Read the model definition and answer for the solid it produces. Units are mm, in the model's axes. A direction names the side the tool comes from. Coordinates: 2 decimals unless noted, no trailing zeros. Order: outer loops, then holes, each group sorted by start corner. A loop starts at its lowest first (then second) coordinate and runs counter-clockwise, first axis right, second up. Notation, with made-up numbers: M 59.25,11 L 91.25,11 A24 ccw 91.25,41 Z; hole C -4,43 d6. An arc over 180 degrees is marked long. One line per question, with ' | ' between items. Start each with the question number.
1) Find section C-C, the plane y = -2. Write down the section's boundary in (x, z).
2) Consider probe 1 along X at (y, z) = (2.5, 0); probe 2 along Y at (x, z) = (0, 0.25); probe 3 along Y at (x, z) = (2.5, 2.25). Determine where each line is inside the solid, lowest interval first.
3) The mould has two halves that part along X. Classify faces 1 (the face through (1, 11.79, -1)), 2 (the face through (0, 11, -2.5)), 3 (the face through (1.151, 9.459, -1.502)): +X half, -X half, draft (parallel to the pull), parting line (faces both ways), or undercut.
4) Given P1, Ø1.6, axis at y = 10.5, z = 1, coming from the -X side; P2, Ø2, axis at x = 0.5, y = 4.5, coming from the -Z side; P3, Ø3, axis at x = 0.5, z = 2, coming from the +Y side; P4, Ø1.3, axis at x = 0, y = 11, coming from the -Z side, each flat-ended and moving along its own axis, determine where each tip first touches the part or whether it passes through.
5) Find section A-A, the plane x = 0. Write down the section's boundary in (y, z), plus the area to 3 significant figures.
6) A tool of negligible diameter and unlimited length cuts with its end or side. For faces 4 (the face through (-0.6, 11, -2)), 5 (the face through (0, -18.01, 0)), 6 (the face through (-0.541, -4.349, 1.717)), from which of +Z, -Z, +X, -X, +Y, -Y can it reach the whole face along a straight path? Write none if from no direction.
7) Find section B-B, the plane z = 0. Write down the section's boundary in (x, y), plus the area to 3 significant figures.
from build123d import *

# Parameters (mm, degrees)
CUT_EXTRUDE1_DEPTH = 1.43


with BuildPart() as part:
    # Sketch1 → Revolve1 (revolve)
    with BuildSketch(Plane(origin=(0, 0, 0), x_dir=(0, 0, -1), z_dir=(1, 0, 0))):
        Polygon((0, 11.789679649), (-3.7, 11.789679649), (-1.8, 9.339679649), (-1.8, -17.660320351), (-1.528571429, -18.010320351), (0, -18.010320351), align=None)
    revolve(axis=Axis((0, 14.440515102, 0), (0, -1, 0)))

    # Sketch2 → Cut-Extrude1 (cut)
    with BuildSketch(Plane(origin=(0, 11.789679649, 0), x_dir=(1, 0, 0), z_dir=(0, 1, 0))):
        Polygon((2.5, -0.6), (0.6, -0.6), (0.6, -2.5), (-0.6, -2.5), (-0.6, -0.6), (-2.5, -0.6), (-2.5, 0.6), (-0.6, 0.6), (-0.6, 2.5), (0.6, 2.5), (0.6, 0.6), (2.5, 0.6), align=None)
    extrude(amount=-CUT_EXTRUDE1_DEPTH, mode=Mode.SUBTRACT)


solid = part.part
Report:
1) outline: C 0,0 d3.6
2) probe 1: x = -1.8 to 1.8 | probe 2: y = -18.01 to 10.36 | probe 3: y = 11.36 to 11.79
3) face 1: draft | face 2: undercut | face 3: parting line
4) P1: stops at x = -3.2 | P2: stops at z = -1.8 | P3: stops at y = 11.79 | P4: stops at z = -3.59
5) outline: M -18.01,-1.53 L -17.66,-1.8 L 9.34,-1.8 L 11.79,-3.7 L 11.79,-2.5 L 10.36,-2.5 L 10.36,2.5 L 11.79,2.5 L 11.79,3.7 L 9.34,1.8 L -17.66,1.8 L -18.01,1.53 Z | area: 105 mm^2
6) face 4: +Y | face 5: +Z, -Z, +X, -X, -Y | face 6: -Y
7) outline: M -3.7,11.79 L -1.8,9.34 L -1.8,-17.66 L -1.53,-18.01 L 1.53,-18.01 L 1.8,-17.66 L 1.8,9.34 L 3.7,11.79 L 2.5,11.79 L 2.5,10.36 L -2.5,10.36 L -2.5,11.79 Z | area: 105 mm^2
